from build123d import *

# Parameters (mm, degrees)
SKETCH1_R               = 6.477
BOSS_EXTRUDE2_DEPTH     = 12.7
CUT_EXTRUDE2_DEPTH      = 2.032
CUT_EXTRUDE2_TAPER      = 15
SKETCH4_OUTSIDE_W       = 47.17
SKETCH4_OUTSIDE_H       = 39.55
SKETCH4_OUTSIDE_R       = 10.16
CUT_EXTRUDE1_DEPTH      = 112.76
CUT_EXTRUDE1_DEPTH_BACK = 11.16


with BuildPart() as part:
    # Sketch1 → Boss-Extrude2 (new body)
    with BuildSketch(Plane.XY):
        with BuildLine():
            Line((-10.16, 0), (-10.16, 12.7))
            Line((-10.16, 12.7), (-3.302, 28.175956627))
            Line((-3.302, 28.175956627), (-3.302, 91.991545598))
            ThreePointArc((-3.302, 91.991545598), (0, 111.76), (3.302, 91.991545598))
            Line((3.302, 91.991545598), (3.302, 28.175956627))
            Line((3.302, 28.175956627), (10.16, 12.7))
            Line((10.16, 12.7), (10.16, 0))
            ThreePointArc((10.16, 0), (0, -10.16), (-10.16, 0))
        make_face()
        Circle(SKETCH1_R, mode=Mode.SUBTRACT)
        with Locations((0, 101.6)):
            Circle(SKETCH1_R, mode=Mode.SUBTRACT)
    extrude(amount=-BOSS_EXTRUDE2_DEPTH)

    # Sketch3 → Cut-Extrude2 (cut)
    with BuildSketch(Plane.XY):
        with BuildLine():
            ThreePointArc((-0.508, 89.408), (-1.585630735, 88.961630735), (-2.032, 87.884))
            Line((-2.032, 87.884), (-2.032, 32.766))
            ThreePointArc((-2.032, 32.766), (-1.585630735, 31.688369265), (-0.508, 31.242))
            Line((-0.508, 31.242), (0.508, 31.242))
            ThreePointArc((0.508, 31.242), (1.585630735, 31.688369265), (2.032, 32.766))
            Line((2.032, 32.766), (2.032, 87.884))
            ThreePointArc((2.032, 87.884), (1.585630735, 88.961630735), (0.508, 89.408))
            Line((0.508, 89.408), (-0.508, 89.408))
        make_face()
    cut_extrude2 = extrude(amount=-CUT_EXTRUDE2_DEPTH, taper=CUT_EXTRUDE2_TAPER, mode=Mode.SUBTRACT)

    # Mirror1: Cut-Extrude2 across plane
    add(cut_extrude2.mirror(Plane.XY.offset(-6.35)), mode=Mode.SUBTRACT)

    # Sketch4 outside → Cut-Extrude1 (cut, two sides)
    with BuildSketch(Plane(origin=(0, 0, 0), x_dir=(1, 0, 0), z_dir=(0, 1, 0))) as cut_extrude1_sk:
        with Locations((0, 6.35)):
            Rectangle(SKETCH4_OUTSIDE_W, SKETCH4_OUTSIDE_H)
        with Locations((0, 6.16880724)):
            Circle(SKETCH4_OUTSIDE_R, mode=Mode.SUBTRACT)
    extrude(amount=CUT_EXTRUDE1_DEPTH, mode=Mode.SUBTRACT)
    extrude(cut_extrude1_sk.sketch, amount=-CUT_EXTRUDE1_DEPTH_BACK, mode=Mode.SUBTRACT)


solid = part.part
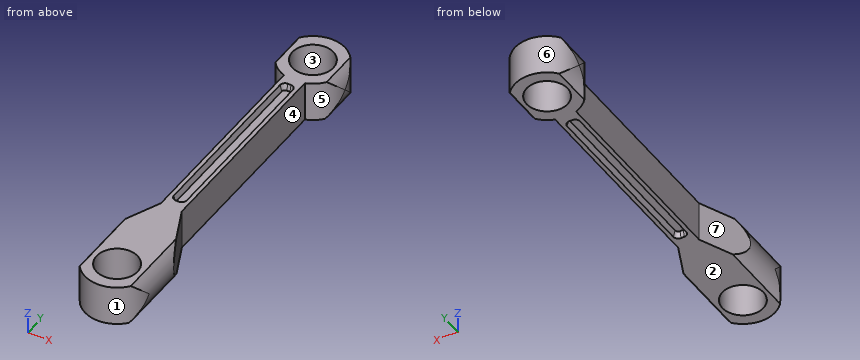
Geometry: final body of the model. Coordinates: model frame, mm. Face numbers are marked on the shaded views. A direction names the side the tool comes from. Give positions to 0.01 mm unless a question says otherwise; leave off trailing zeros. Write each loop counter-clockwise with the first axis right and the second up, starting at its lowest first coordinate (ties: lowest second). Pieces come first, ordered by that corner, then holes. Notation, with made-up numbers: (-8.5, 20) - (24.5, 20) arc R23 ccw to (24.5, 53) - close; hole circle Ø10 at (82, 52.5). An arc over 180 degrees is marked (long way). Return JSON: item names as keys, results as strings. Group by question number.
1) Section A-A on y = 3.5. Return the cut outline in (x, z).
2) Section C-C on y = 25. Return the cut outline in (x, z).
3) First-contact query: P1, Ø1.5, axis at x = 0, y = 65.5, coming from the -Z side; P2, Ø2, axis at y = 46, z = -2.5, coming from the -X side; P3, Ø6.5, axis at y = 60.5, z = -7.5, coming from the +X side. Flat tips, straight axial feed; report the tip coordinate or a pass-through.
4) Set-up query: the marked faces 5, 6 and 7. Return all of +Z, -Z, +X, -X, +Y, -Y with unobstructed straight access to the full face (end or side cutting, diameter ignored); none if empty.
5) Mould query, pull axis X, two halves, no side actions, for the marked faces 1, 2, 3 and 4. Classes: released by +X, released by -X, zero draft, split by the parting line, or undercut.
6) Line query: line 1 (Y direction, x = 0, z = -7.75); line 2 (Y direction, x = -4.25, z = -7.5); line 3 (Y direction, x = 3.5, z = -2.5). Output: solid intervals per line, ascending.
7) Section B-B on z = -9. Return the cut outline in (x, y), plus the area to 3 significant figures.
Filled in:
{
 "1": {"outline": "(-8.07, 0) arc R10.16 ccw to (-7.78, -12.7) - (-5.45, -12.7) - (-5.45, 0) - close; (5.45, -12.7) - (7.78, -12.7) arc R10.16 ccw to (8.07, 0) - (5.45, 0) - close"},
 "2": {"outline": "(-4.71, -12.7) - (4.71, -12.7) - (4.71, 0) - (-4.71, 0) - close"},
 "3": {"P1": "stops at z = -10.67", "P2": "stops at x = -3.3", "P3": "stops at x = 3.3"},
 "4": {"face 5": "+Z, -Z, +X", "face 6": "+Z, -Z", "face 7": "+Z, -Z, -X"},
 "5": {"face 1": "split by the parting line", "face 2": "zero draft", "face 3": "undercut", "face 4": "released by +X"},
 "6": {"line 1": "y = -10.16 to -6.48, 6.48 to 95.12, 108.08 to 111.76", "line 2": "y = -9.23 to -4.89, 4.89 to 26.04, 92.37 to 96.71, 106.49 to 110.83", "line 3": "y = -9.54 to -5.45, 5.45 to 27.73, 92.06 to 96.15, 107.05 to 111.14"},
 "7": {"outline": "(-9.76, -2.83) arc R10.16 ccw to (9.76, -2.83) - (9.76, 13.61) - (3.3, 28.18) - (3.3, 91.99) arc R10.16 ccw to (9.76, 98.77) - (9.76, 104.43) arc R10.16 ccw to (-9.76, 104.43) - (-9.76, 98.77) arc R10.16 ccw to (-3.3, 91.99) - (-3.3, 28.18) - (-9.76, 13.61) - close; hole circle Ø12.95 at (0, 0); hole circle Ø12.95 at (0, 101.6)", "area": "1,090 mm^2"}
}
